from build123d import *

# Parameters (mm, degrees)
SKICA1_W                 = 101
SKICA1_H                 = 33
P_IDAT_VYSUNUT_M1_DEPTH  = 30
SKICA2_W                 = 50
SKICA2_H                 = 65
P_IDAT_VYSUNUT_M2_DEPTH  = 30
P_IDAT_VYSUNUT_M3_DEPTH  = 50
ODEBRAT_VYSUNUT_M5_DEPTH = 18.9
SKICA17_R                = 2.8
ODEBRAT_VYSUNUT_M6_DEPTH = 14.2
SKICA18_R                = 7.5
ODEBRAT_VYSUNUT_M7_DEPTH = 8.7


with BuildPart() as part:
    # Skica1 → Přidat vysunutím1 (new body)
    with BuildSketch(Plane.XY):
        with Locations((50.5, 16.5)):
            Rectangle(SKICA1_W, SKICA1_H)
    extrude(amount=P_IDAT_VYSUNUT_M1_DEPTH)

    # Skica2 → Přidat vysunutím2 (add)
    with BuildSketch(Plane.XY.offset(30)):
        with Locations((50.25, -16)):
            Rectangle(SKICA2_W, SKICA2_H)
    extrude(amount=P_IDAT_VYSUNUT_M2_DEPTH)

    # Skica3 → Přidat vysunutím3 (add)
    with BuildSketch(Plane.ZY.offset(-25.25)):
        Polygon((30, 33), (60, 16.5), (30, 16.5), align=None)
    extrude(amount=-P_IDAT_VYSUNUT_M3_DEPTH)

    # Skica6 → Odebrat vysunutím5 (cut)
    with BuildSketch(Plane.XY.offset(60)):
        Polygon((29.945, 15.35), (70.555, 15.35), (72.85, -47.35), (27.65, -47.35), align=None)
    extrude(amount=-ODEBRAT_VYSUNUT_M5_DEPTH, mode=Mode.SUBTRACT)

    # Skica17 → Odebrat vysunutím6 (cut)
    with BuildSketch(Plane.XY.offset(41.1)):
        with Locations((50.144115431, -17.85)):
            Circle(SKICA17_R)
    extrude(amount=-ODEBRAT_VYSUNUT_M6_DEPTH, mode=Mode.SUBTRACT)

    # Skica18 → Odebrat vysunutím7 (cut)
    with BuildSketch(Plane(origin=(0, 0, 30), x_dir=(-1, 0, 0), z_dir=(0, 0, -1))):
        with Locations((-50.144115431, -17.85)):
            Circle(SKICA18_R)
    extrude(amount=-ODEBRAT_VYSUNUT_M7_DEPTH, mode=Mode.SUBTRACT)


solid = part.part
Input: part model. Units: mm. Frame: model coordinates. A direction names the side the tool comes from. Coordinates: 2 decimals unless noted, no trailing zeros. Order: outer loops, then holes, each group sorted by start corner. A loop starts at its lowest first (then second) coordinate and runs counter-clockwise, first axis right, second up.
1. Ray query, line 1 along X through (y, z) = (7, 38); line 2 along Z through (x, y) = (45.5, -10); line 3 along Y through (x, z) = (6.5, 11). Return the intervals inside material, ascending.
Checked values:
line 1: x = 25.25 to 75.25
line 2: z = 30 to 41.1
line 3: y = 0 to 33
2. Contact query for flat-ended pins moving along their axis: P1, Ø24, axis at x = 50.14, y = -17.85, coming from the -Z side; P2, Ø5, axis at x = 73.5, z = 22, coming from the -Y side; P3, Ø5.5, axis at x = 60.5, z = 54, coming from the +Y side; P4, Ø8, axis at y = -30.5, z = 24.5, coming from the -X side. Output: stop coordinate, or through.
Checked values:
P1: stops at z = 30
P2: stops at y = 0
P3: stops at y = 21.31
P4: passes through
3. Cut plane C-C, the plane x = 74. Return loops of the section in (y, z), plus the area to 3 significant figures.
Checked values:
outline: (-48.5, 30) - (0, 30) - (0, 0) - (33, 0) - (33, 30) - (16.5, 60) - (-48.5, 60) - close
area: 3,190 mm2
4. Cut plane B-B, the plane z = 49.5. Return loops of the section in (x, y) (3 decimals), plus the area to 3 significant figures.
Checked values:
outline: (25.25, -48.5) - (75.25, -48.5) - (75.25, 22.275) - (25.25, 22.275) - close; hole (27.65, -47.35) - (72.85, -47.35) - (70.555, 15.35) - (29.945, 15.35) - close
area: 849 mm2
5. Draft query along X for faces 1 (the flat face through (56, -16, 41.1)), 2 (the cylindrical face through (47.347, -17.727, 39.917)), 3 (the flat face through (101, 16, 15)), 4 (the flat face through (28, -9, 60)). Return one class per face: +X half, -X half, draft (parallel to the pull), parting line (faces both ways), or undercut.
Checked values:
face 1: undercut
face 2: undercut
face 3: +X half
face 4: draft
6. Cut plane D-D, the plane y = -28. Return loops of the section in (x, z).
Checked values:
outline: (25.25, 30) - (75.25, 30) - (75.25, 60) - (72.14, 60) - (72.14, 41.1) - (28.36, 41.1) - (28.36, 60) - (25.25, 60) - close
7. Access query for faces 5 (the flat face through (50, -21, 38.7)), 6 (the flat face through (88, 17, 30)), 7 (the flat face through (50, 15.35, 51)). Directions: +Z, -Z, +X, -X, +Y, -Y. A direction counts if a zero-diameter tool reaches every point of the face in a straight line with its end or side. Return the directions, or none.
Checked values:
face 5: -Z
face 6: +Z, +X, +Y, -Y
face 7: +Z
8. Cut plane A-A, the plane y = -17.85. Return loops of the section in (x, z), plus the area to 3 significant figures.
Checked values:
outline: (25.25, 30) - (42.64, 30) - (42.64, 38.7) - (47.34, 38.7) - (47.34, 41.1) - (28.73, 41.1) - (28.73, 60) - (25.25, 60) - close; (52.94, 38.7) - (57.64, 38.7) - (57.64, 30) - (75.25, 30) - (75.25, 60) - (71.77, 60) - (71.77, 41.1) - (52.94, 41.1) - close
area: 543 mm2
